Check sheet for the drawn part. Datum: minimum x, y, z corner. Units: mm. A direction names the side the tool comes from. Coordinates: 2 decimals unless noted, no trailing zeros. Loops run counter-clockwise (first coordinate to the right, second up) from the corner with the lowest first, then second, coordinate; pieces in that order, holes last. Notation, with made-up numbers: M 10.5,51.25 L 40.5,51.25 A28 ccw 40.5,87.25 Z; hole C 5.25,85.5 d5. An arc over 180 degrees is marked long. Use CSV: the item, a comma, the result in double quotes. Start each with the question number.
(1) Section check D-D on y = 43. Record the cut outline in (x, z), and give its area (3 significant figures).
(2) Scan lines: line 1 (Z direction, x = 55.5, y = 19.5); line 2 (Z direction, x = 26.5, y = 45.5); line 3 (X direction, y = 44, z = 23.5). Record each from-to range of solid material in increasing order.
(3) Go/stop test with flat-tipped pins: pin 1 Ø4 at (x, y) = (52, 12) entering from +Z; pin 2 Ø11 at (x, y) = (32, 42.5) entering from +Z; pin 3 Ø10 at (y, z) = (14, 18) entering from +X; pin 4 Ø10 at (y, z) = (10, 21) entering from +X. Record where each tip stops, or that it passes through.
(4) Section check B-B on z = 16.5. Record the cut outline in (x, y), and give its area (3 significant figures).
(5) Section check C-C on x = 8. Record the cut outline in (y, z), and give its area (3 significant figures).
(6) Draft check along X on the marked faces 4, 5, 6 and 7. Enter one of: pulls with the +X half, pulls with the -X half, needs draft (parallel to the pull), parting line crosses it, or undercut.
(7) Set-up check for the marked faces 1, 2 and 3: record each of +Z, -Z, +X, -X, +Y, -Y from which the full face is reachable in a straight line by a thin tool's end or side.
(8) Section check A-A on y = 10.5. Record the cut outline in (x, z), and give its area (4 significant figures).
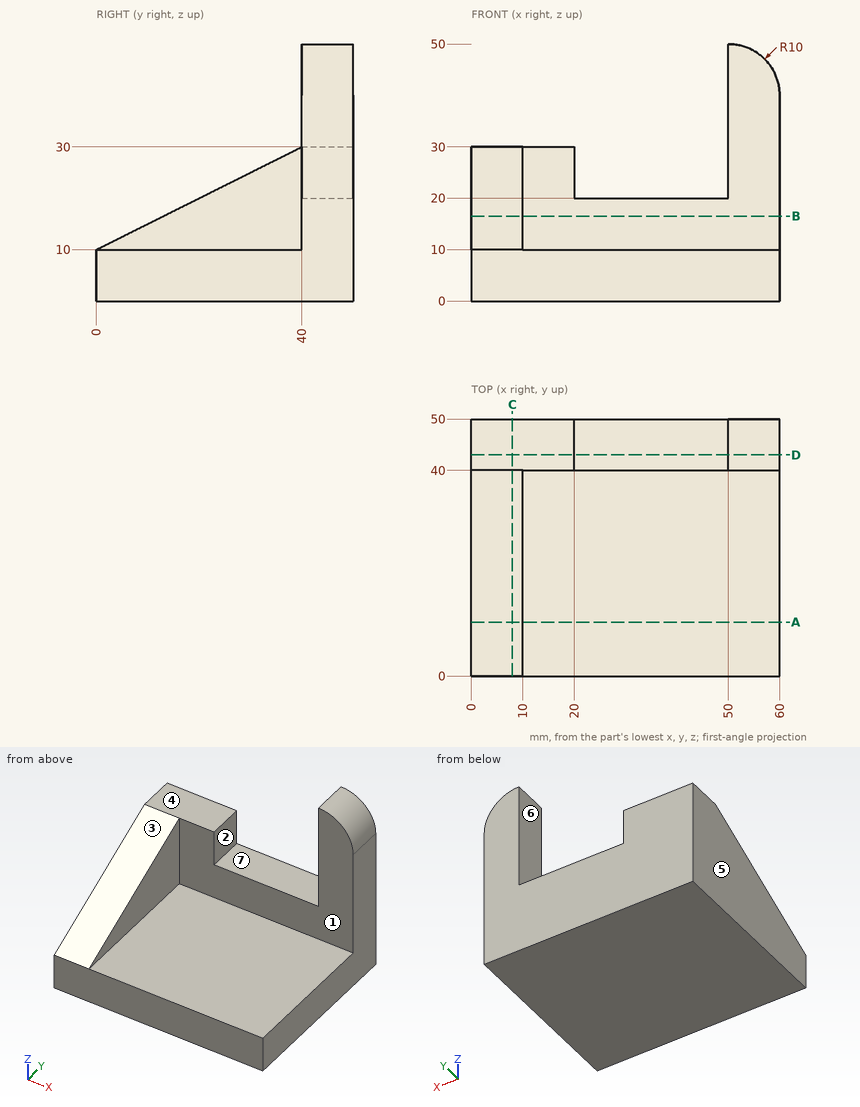
Outcome:
1,outline,"M 0,0 L 60,0 L 60,40 A10 ccw 50,50 L 50,20 L 20,20 L 20,30 L 0,30 Z"
1,area,"1,680 mm²"
2,line 1,"z = 0 to 10"
2,line 2,"z = 0 to 20"
2,line 3,"x = 0 to 20, 50 to 60"
3,pin 1,"stops at z = 10"
3,pin 2,"stops at z = 20"
3,pin 3,"stops at x = 10"
3,pin 4,"passes through"
4,outline,"M 0,13 L 10,13 L 10,40 L 60,40 L 60,50 L 0,50 Z"
4,area,"870 mm²"
5,outline,"M 0,0 L 50,0 L 50,30 L 40,30 L 0,10 Z"
5,area,"1,100 mm²"
6,face 4,"needs draft"
6,face 5,"pulls with the -X half"
6,face 6,"undercut"
6,face 7,"undercut"
7,face 1,"+Z, +X, -Y"
7,face 2,"+Z, +Y, -Y"
7,face 3,"+Z, +X, -X, -Y"
8,outline,"M 0,0 L 60,0 L 60,10 L 10,10 L 10,15.25 L 0,15.25 Z"
8,area,"652.5 mm²"
